Autodesk Inventor part; units mm, degrees
ref_plane "YZ Plane" through (0, 0, 0) normal (1, 0, 0) x (0, 1, 0)
ref_plane "XZ Plane" through (0, 0, 0) normal (0, 1, 0) x (-1, 0, 0)
ref_plane "XY Plane" through (0, 0, 0) normal (0, 0, 1) x (1, 0, 0)
ref_plane "Work Plane1" through (7.2648, 18.7113, 1.7167) normal (0, 0, 1) x (1, 0, 0)
sketch "Sketch1" plane through (7.2648, 18.7113, 1.7167) normal (0, 0, 1) x (1, 0, 0)
  circle A0 centre (-12.9413, -0.2667) radius 7.9502
  line L0 (-5.933, 4.5118) -> (5.37, 4.5118)
  line L1 (5.37, 9.0584) -> (-5.933, 9.0584)
  line L2 (5.37, 9.0584) -> (-5.933, 9.0584)
  circle A1 centre (-12.9413, -0.2667) radius 7.9502
  circle A2 centre (12.9413, -0.2667) radius 7.9502
  line L3 (22.7457, -10.1981) -> (22.7457, 10.1981)
  line L4 (22.7457, 10.1981) -> (-22.7457, 10.1981)
  line L5 (-22.7457, -10.1981) -> (22.7457, -10.1981)
  line L6 (-22.7457, 10.1981) -> (-22.7457, -10.1981)
  line L7 (-5.933, 6.444) -> (-5.933, 4.5118)
  line L8 (-5.933, 9.0584) -> (-5.933, 7.1262)
  line L9 (5.37, 4.5118) -> (5.37, 9.0584)
  line L10 (-5.933, 9.0584) -> (-5.933, 4.5118)
  circle A3 centre (-12.9413, -0.2667) radius 8.25
  circle A4 centre (12.9413, -0.2667) radius 8.25
  point P0 (-7.2648, -18.7113)
  dimension "d5" = 16.5
  dimension "d6" = 16.5
extrude "Extrusion1" add sketch "Sketch1" along normal blind 4 contours L5 L6 L4 L3 | A3 | A4
sketch "Sketch2" plane through (7.2648, 18.7113, 5.7167) normal (0, 0, 1) x (1, 0, 0)
  line L0 (22.7457, -10.1981) -> (22.7457, 10.1981)
  line L1 (22.7457, 10.1981) -> (27.7457, 10.1981)
  line L2 (27.7457, 10.1981) -> (27.7457, -10.1981)
  line L3 (27.7457, -10.1981) -> (22.7457, -10.1981)
  line L4 (22.7457, -10.1981) -> (22.7457, 10.1981)
  line L5 (24.7457, 10.1981) -> (24.7457, -10.1981)
  point P0 (-7.2648, -18.7113)
  dimension "d7" = 5
  dimension "d8" = 2
extrude "Extrusion3" add sketch "Sketch2" against normal blind 30 contours L5 L1 L2 L3
sketch "Sketch3" plane through (7.2648, 18.7113, 5.7167) normal (0, 0, 1) x (1, 0, 0)
  line L0 (22.7457, -10.1981) -> (22.7457, 10.1981)
  line L1 (24.7457, -10.1981) -> (24.7457, 10.1981)
  line L2 (22.7457, 10.1981) -> (24.7457, 10.1981)
  line L3 (24.7457, 10.1981) -> (24.7457, -10.1981)
  line L4 (24.7457, -10.1981) -> (22.7457, -10.1981)
  line L5 (22.7457, -10.1981) -> (22.7457, 10.1981)
  point P0 (-7.2648, -18.7113)
extrude "Extrusion4" add sketch "Sketch3" against normal blind 4
sketch "Sketch4" plane through (-15.4809, 28.9094, 5.7167) normal (0, 1, 0) x (1, 0, 0)
  line L0 (50.4914, 0) -> (50.4914, 30)
  line L1 (50.4914, 30) -> (62.668, 0)
  line L2 (62.668, 0) -> (60.736, 0)
  line L3 (60.736, 0) -> (50.4914, 25.24)
  line L4 (55.6137, 0) -> (50.4914, 13.4027)
  line L5 (53.764, 0) -> (50.4914, 8.0628)
  line L6 (50.4914, 13.4027) -> (50.4914, 8.0628)
  line L7 (53.764, 0) -> (55.6137, 0)
  point P0 (15.4809, 5.7167)
extrude "Extrusion5" add sketch "Sketch4" against normal blind 5
sketch "Sketch5" plane through (-15.4809, 8.5132, 1.7167) normal (0, -1, 0) x (1, 0, 0)
  line L0 (50.4914, -26) -> (50.4914, -21.24)
  line L1 (50.4914, -26) -> (62.668, 4)
  line L2 (62.668, 4) -> (60.736, 4)
  line L3 (60.736, 4) -> (50.4914, -21.24)
  line L4 (50.4914, -9.4027) -> (50.4914, -4.0628)
  line L5 (50.4914, -9.4027) -> (55.6137, 4)
  line L6 (55.6137, 4) -> (53.764, 4)
  line L7 (53.764, 4) -> (50.4914, -4.0628)
  point P0 (15.4809, -1.7167)
extrude "Extrusion6" add sketch "Sketch5" against normal blind 5
properties part number "USsensor holder"
Check sheet for the modelled part. Datum: model origin and axes. Units: mm. A direction names the side the tool comes from. Coordinates: 2 decimals unless noted, no trailing zeros. Write each loop counter-clockwise with the first axis right and the second up, starting at its lowest first coordinate (ties: lowest second). Pieces come first, ordered by that corner, then holes.
Item 1: Mould release check, pull along Y, two halves, no side actions. Record for faces 5 (the face through (39, 11, 5.717)), 6 (the face through (7, 23.223, 4)): released by +Y, released by -Y, zero draft, split by the parting line, or undercut.
Numbers:
face 5: zero draft
face 6: undercut
Item 2: Cross-section at B-B on x = 7.5. Record the boundary of the cut face in (y, z), then the cut area to 3 significant figures.
Numbers:
outline: (8.51, 1.72) - (23.22, 1.72) - (23.22, 5.72) - (8.51, 5.72) - close; (27.77, 1.72) - (28.91, 1.72) - (28.91, 5.72) - (27.77, 5.72) - close
area: 63.4 mm2
Item 3: Cross-section at A-A on z = 3.25. Record the boundary of the cut face in (x, y), then the cut area to 3 significant figures.
Numbers:
outline: (-15.48, 8.51) - (35.01, 8.51) - (35.01, 28.91) - (-15.48, 28.91) - close; (37.28, 8.51) - (39.19, 8.51) - (39.19, 13.51) - (37.28, 13.51) - close; (37.28, 23.91) - (39.19, 23.91) - (39.19, 28.91) - (37.28, 28.91) - close; (44.25, 8.51) - (46.19, 8.51) - (46.19, 13.51) - (44.25, 13.51) - close; (44.25, 23.91) - (46.19, 23.91) - (46.19, 28.91) - (44.25, 28.91) - close; hole circle Ø15.9 at (-5.68, 18.44); hole (1.33, 23.22) - (12.63, 23.22) - (12.63, 27.77) - (1.33, 27.77) - close; hole circle Ø15.9 at (20.21, 18.44)
area: 620 mm2
Item 4: Access from +Z, -Z, +X, -X, +Y, -Y to the whole of each face (thin tool, end or side, straight path). Record for faces 1 (the face through (7, 27.77, 4)), 2 (the face through (32.01, 19, -11)), 3 (the face through (40.205, 10.978, -6.727)), 4 (the face through (37, 23.909, 0)).
Numbers:
face 1: +Z, -Z
face 2: -Z, -X, +Y, -Y
face 3: +Y, -Y
face 4: +Z, -Z, +X
Item 5: Scan lines: probe 1 along X at (y, z) = (11.5, 2.25); probe 2 along X at (y, z) = (26, 1.25); probe 3 along X at (y, z) = (12.75, 3.5). Record each from-to range of solid material in increasing order.
Numbers:
probe 1: x = -15.48 to -9.55, -1.81 to 16.34, 24.08 to 35.01, 36.88 to 38.81, 43.85 to 45.78
probe 2: x = 32.01 to 35.01, 36.47 to 38.43, 43.44 to 45.37
probe 3: x = -15.48 to -11.22, -0.13 to 14.66, 25.75 to 35.01, 37.38 to 39.29, 44.36 to 46.29
Item 6: Depth check by flat-ended pin: pin 1 Ø12 at (y, z) = (19.5, -2.5) entering from -X; pin 2 Ø5 at (x, y) = (-9, 24.5) entering from -Z; pin 3 Ø5 at (y, z) = (22.5, -14) entering from -X; pin 4 Ø2 at (y, z) = (25, 3.5) entering from +X. Enter the tip coordinate at first touch or a pass-through.
Numbers:
pin 1: stops at x = -15.48
pin 2: stops at z = 1.72
pin 3: stops at x = 32.01
pin 4: stops at x = 46.69
Item 7: Cross-section at C-C on y = 24.5. Record the boundary of the cut face in (x, z), then the cut area to 3 significant figures.
Numbers:
outline: (-15.48, 1.72) - (-10.83, 1.72) - (-10.83, 5.72) - (-15.48, 5.72) - close; (-0.53, 1.72) - (1.33, 1.72) - (1.33, 5.72) - (-0.53, 5.72) - close; (12.63, 1.72) - (15.05, 1.72) - (15.05, 5.72) - (12.63, 5.72) - close; (25.36, 1.72) - (32.01, 1.72) - (32.01, -24.28) - (35.01, -24.28) - (47.19, 5.72) - (45.26, 5.72) - (35.01, -19.52) - (35.01, -7.69) - (40.13, 5.72) - (38.28, 5.72) - (35.01, -2.35) - (35.01, 5.72) - (25.36, 5.72) - close
area: 227 mm2
Item 8: Cross-section at D-D on z = -13. Record the boundary of the cut face in (x, y).
Numbers:
outline: (32.01, 8.51) - (35.01, 8.51) - (35.01, 28.91) - (32.01, 28.91) - close; (37.66, 8.51) - (39.59, 8.51) - (39.59, 13.51) - (37.66, 13.51) - close; (37.66, 23.91) - (39.59, 23.91) - (39.59, 28.91) - (37.66, 28.91) - close
